```python
from build123d import *

# Parameters (mm, degrees)
SKETCH1_W           = 5.4
SKETCH1_H           = 15.4
SKETCH1_W_2         = 5
SKETCH1_H_2         = 15
BOSS_EXTRUDE1_DEPTH = 5
SKETCH2_W           = 10
SKETCH2_H           = 25
CUT_EXTRUDE1_DEPTH  = 10


with BuildPart() as part:
    # Sketch1 → Boss-Extrude1 (new body)
    with BuildSketch(Plane.XY):
        Polygon((0, 0), (2.5, 0), (5, 20), (5, 100), (0, 100), (0, 90), (-15, 90), (-15, 65), (0, 65), (0, 44.5), (-15, 44.5), (-15, 19.5), (0, 19.5), align=None)
        with Locations((-7.7, 77.5)):
            Rectangle(SKETCH1_W, SKETCH1_H, mode=Mode.SUBTRACT)
        with Locations((-7.5, 32)):
            Rectangle(SKETCH1_W_2, SKETCH1_H_2, mode=Mode.SUBTRACT)
    extrude(amount=BOSS_EXTRUDE1_DEPTH)

    # Sketch2 → Cut-Extrude1 (cut)
    with BuildSketch(Plane.XY.offset(5)):
        with Locations((-10, 32)):
            Rectangle(SKETCH2_W, SKETCH2_H)
    extrude(amount=-CUT_EXTRUDE1_DEPTH, mode=Mode.SUBTRACT)


solid = part.part
```
Here's how the part is built. I have some questions about the finished solid (model axes, mm). A direction names the side the tool comes from. Give positions to 0.01 mm unless a question says otherwise; leave off trailing zeros. Write each loop counter-clockwise with the first axis right and the second up, starting at its lowest first coordinate (ties: lowest second). Pieces come first, ordered by that corner, then holes.
(1) Thinking about a two-plate mould opening in Y: for faces 1 (the face through (-8, 85.2, 2)), 2 (the face through (-3, 19.5, 2)), 3 (the face through (-15, 78, 2)), which applies, pulls with the +Y half, pulls with the -Y half, needs draft (parallel to the pull), parting line crosses it, or undercut?
Output values:
face 1: undercut
face 2: pulls with the -Y half
face 3: needs draft
(2) If I drill on L1, parallel to Y at x = -3.5, z = 1.55; L2, parallel to X at y = 76, z = 0.3; L3, parallel to Y at x = -9.75, z = 1.85, over which ranges is the centre line in solid material (lowest first)?
Output values:
L1: y = 19.5 to 44.5, 65 to 90
L2: x = -15 to -10.4, -5 to 5
L3: y = 65 to 69.8, 85.2 to 90
(3) Imagine slicing it at A-A, the plane y = 78.5. Write out the boundary of the cut face in (x, z), and give its area (3 significant figures).
Output values:
outline: (-15, 0) - (-10.4, 0) - (-10.4, 5) - (-15, 5) - close; (-5, 0) - (5, 0) - (5, 5) - (-5, 5) - close
area: 73.0 mm2
(4) Will these pins go through, and if not, where does the flat tip stop? pin 1 (1.5 mm diameter, centred on y = 5.5, z = 3.5, fed in from -X); pin 2 (1.5 mm diameter, centred on x = -7, z = 3.5, fed in from +Y); pin 3 (2 mm diameter, centred on x = -9, z = 0.5, fed in from -Y).
Output values:
pin 1: stops at x = 0
pin 2: stops at y = 90
pin 3: stops at y = 65
(5) Imagine slicing it at C-C, the plane z = 1.7. Write out the boundary of the cut face in (x, y), and give its area (3 significant figures).
Output values:
outline: (-15, 65) - (0, 65) - (0, 44.5) - (-5, 44.5) - (-5, 19.5) - (0, 19.5) - (0, 0) - (2.5, 0) - (5, 20) - (5, 100) - (0, 100) - (0, 90) - (-15, 90) - close; hole (-10.4, 69.8) - (-5, 69.8) - (-5, 85.2) - (-10.4, 85.2) - close
area: 892 mm2
(6) Imagine slicing it at B-B, the plane x = -6.5. Write out the boundary of the cut face in (y, z), and give its area (3 significant figures).
Output values:
outline: (65, 0) - (69.8, 0) - (69.8, 5) - (65, 5) - close; (85.2, 0) - (90, 0) - (90, 5) - (85.2, 5) - close
area: 48.0 mm2
(7) Imagine slicing it at D-D, the plane x = -12. Write out the boundary of the cut face in (y, z).
Output values:
outline: (65, 0) - (90, 0) - (90, 5) - (65, 5) - close
(8) On a 3-axis mill with a long thin cutter (end or side, diameter ignored), from which of +Z, -Z, +X, -X, +Y, -Y can I reach the whole of each face in a straight line? I mean faces 4 (the face through (0, 10, 2)), 5 (the face through (-2, 44.5, 2)), 6 (the face through (-10.4, 77, 2)). Say none if no direction works.
Output values:
face 4: +Z, -Z, -X, -Y
face 5: +Z, -Z, -X
face 6: +Z, -Z
